Check sheet for the drawn part. Datum: minimum x, y, z corner. Units: mm. A direction names the side the tool comes from. Coordinates: 2 decimals unless noted, no trailing zeros. Write each loop counter-clockwise with the first axis right and the second up, starting at its lowest first coordinate (ties: lowest second). Pieces come first, ordered by that corner, then holes. Notation, with made-up numbers: (-10, 86.25) - (44, 86.25) arc R22 cw to (44, 120.25) - close; hole circle Ø8 at (-19, 61). An arc over 180 degrees is marked (long way). Write each question's results on one line, items separated by ' | '.
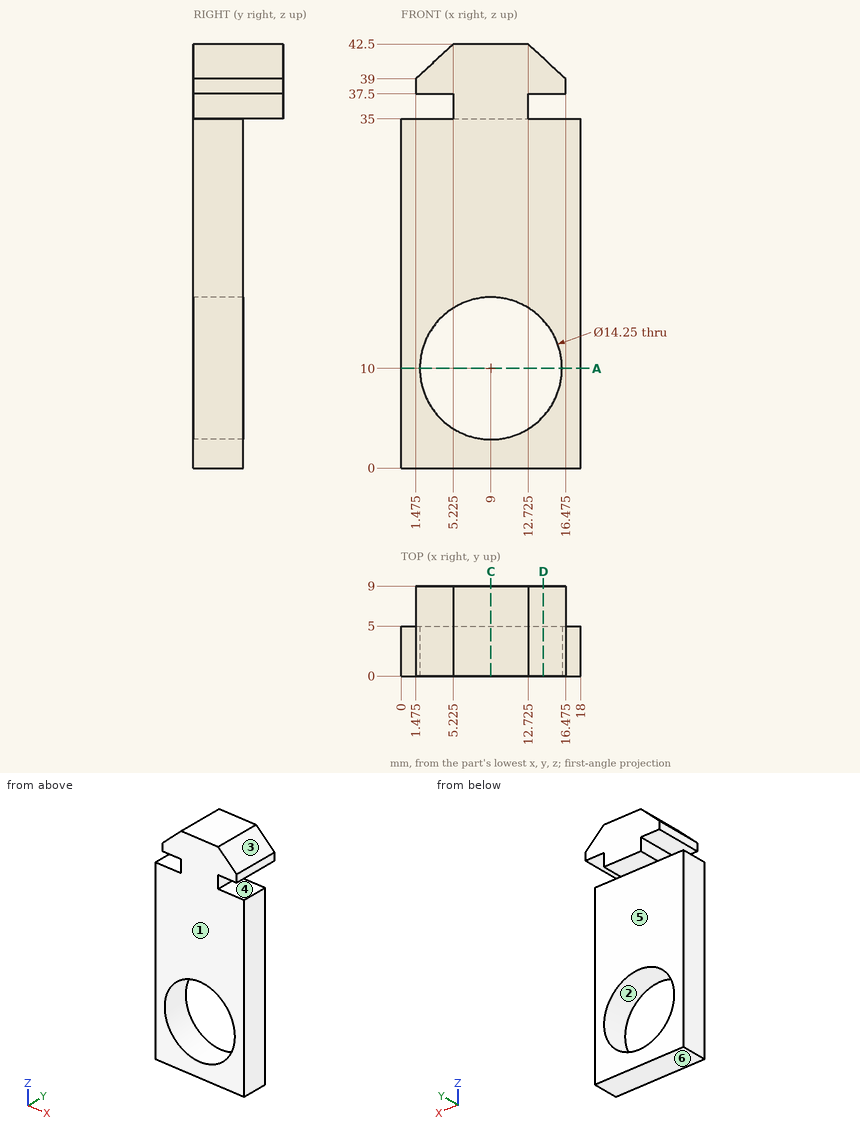
1. Material ranges on L1, parallel to Z at x = 9, y = 2.2 (1 decimal); L2, parallel to Z at x = 14, y = 1.5 (1 decimal); L3, parallel to Y at x = 15.5, z = 27, recorded low to high. Write a range as [from, to].
Values follow:
L1: z = [0, 2.9], [17.1, 42.5] | L2: z = [0, 4.9], [15.1, 35], [37.5, 41.3] | L3: y = [0, 5]
2. Sectioned sample at C-C (x = 9). Record the cut outline in (y, z) (1 decimal).
Values follow:
outline: (0, 0) - (5, 0) - (5, 2.9) - (0, 2.9) - close; (0, 17.1) - (5, 17.1) - (5, 35) - (9, 35) - (9, 42.5) - (0, 42.5) - close
3. Sectioned sample at D-D (x = 14.25). Record the cut outline in (y, z), then the cut area to 3 significant figures.
Values follow:
outline: (0, 0) - (5, 0) - (5, 5.18) - (0, 5.18) - close; (0, 14.82) - (5, 14.82) - (5, 35) - (0, 35) - close; (0, 37.5) - (9, 37.5) - (9, 41.08) - (0, 41.08) - close | area: 159 mm^2
4. Access from +Z, -Z, +X, -X, +Y, -Y to the whole of each face (thin tool, end or side, straight path). Record for the marked faces 4, 5 and 6.
Values follow:
face 4: +X, +Y, -Y | face 5: -Z, +X, -X, +Y | face 6: -Z, +X, -X, +Y, -Y
5. Go/stop test with flat-tipped pins: pin 1 (1.5 mm diameter, centred on y = 7, z = 15.5, fed in from +X); pin 2 (0.8 mm diameter, centred on y = 3.5, z = 38.5, fed in from -X) (1 decimal); pin 3 (1.9 mm diameter, centred on x = 15.5, y = 6, fed in from -Z); pin 4 (1.2 mm diameter, centred on y = 4, z = 36, fed in from +X) (1 decimal). Record where each tip stops, or that it passes through.
Values follow:
pin 1: passes through | pin 2: stops at x = 1.5 | pin 3: stops at z = 37.5 | pin 4: stops at x = 12.7
6. Draft check along X on the marked faces 1, 2 and 3. Enter one of: pulls with the +X half, pulls with the -X half, needs draft (parallel to the pull), parting line crosses it, or undercut.
Values follow:
face 1: needs draft | face 2: undercut | face 3: pulls with the +X half
7. Sectioned sample at A-A (z = 10). Record the cut outline in (x, y) (1 decimal).
Values follow:
outline: (0, 0) - (1.9, 0) - (1.9, 5) - (0, 5) - close; (16.1, 0) - (18, 0) - (18, 5) - (16.1, 5) - close
